Source: three-view drawing plus pictorial views. Frame: mm from the lowest corner of the part. Give positions to 0.01 mm unless a question says otherwise; leave off trailing zeros. Loops run counter-clockwise (first coordinate to the right, second up) from the corner with the lowest first, then second, coordinate; pieces in that order, holes last.
1. First-contact query: P1, Ø2, axis at x = 44, z = 13.5, coming from the -Y side. Flat tip, straight axial feed; report the tip coordinate or a pass-through.
2. Section B-B, the plane y = 2.5. Output: boundary loops of the cut face in (x, z).
3. Section C-C, the plane z = 14.5. Output: boundary loops of the cut face in (x, y).
4. Material intervals for line 1 along Z through (x, y) = (134, 2); line 2 along Y through (x, z) = (102.5, 10.5), sorted ascending.
5. Section A-A, the plane x = 109. Output: boundary loops of the cut face in (y, z), then the cut area to 3 significant figures.
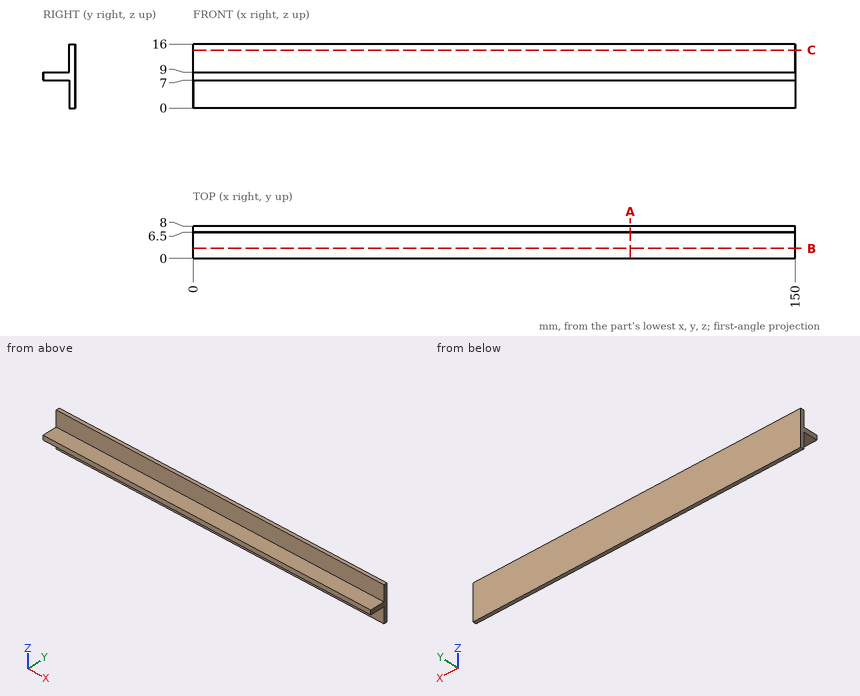
Answers below:
1. P1: stops at y = 6.5
2. outline: (0, 7) - (150, 7) - (150, 9) - (0, 9) - close
3. outline: (0, 6.5) - (150, 6.5) - (150, 8) - (0, 8) - close
4. line 1: z = 7 to 9
4. line 2: y = 6.5 to 8
5. outline: (0, 7) - (6.5, 7) - (6.5, 0) - (8, 0) - (8, 16) - (6.5, 16) - (6.5, 9) - (0, 9) - close
5. area: 37.0 mm2
